```python
from build123d import *

# Parameters (mm, degrees)
SKETCH1_W           = 42
SKETCH1_H           = 14
SKETCH1_R           = 2.75
BOSS_EXTRUDE1_DEPTH = 12.7
SKETCH2_W           = 7
SKETCH2_H           = 1.27
CUT_EXTRUDE1_DEPTH  = 14


with BuildPart() as part:
    # Sketch1 → Boss-Extrude1 (new body)
    with BuildSketch(Plane(origin=(0, 0, 0), x_dir=(1, 0, 0), z_dir=(0, 1, 0))):
        Rectangle(SKETCH1_W, SKETCH1_H)
        with Locations((-16, 0)):
            Circle(SKETCH1_R, mode=Mode.SUBTRACT)
        with Locations((16, 0)):
            Circle(SKETCH1_R, mode=Mode.SUBTRACT)
    extrude(amount=BOSS_EXTRUDE1_DEPTH)

    # Sketch2 → Cut-Extrude1 (cut)
    with BuildSketch(Plane.XY.offset(7)):
        with Locations((0, 0.635)):
            Rectangle(SKETCH2_W, SKETCH2_H)
    extrude(amount=-CUT_EXTRUDE1_DEPTH, mode=Mode.SUBTRACT)


solid = part.part
```
The listing builds one solid part. Answer for the finished solid, in the listing's coordinates (mm). A direction names the side the tool comes from. Coordinates: 2 decimals unless noted, no trailing zeros. Loops run counter-clockwise (first coordinate to the right, second up) from the corner with the lowest first, then second, coordinate; pieces in that order, holes last. Notation, with made-up numbers: (-7, 40.25) -> (48, 40.25) arc R29 cw to (48, 75.25) -> close; hole circle Ø2 at (78, -22.75). An arc over 180 degrees is marked (long way). Use one line per item in the form item = value. Start each with the question number.
Item 1: Flat-ended cylindrical pins translate along their axes: pin 1 Ø3.5 at (x, z) = (1, -3.5) entering from -Y; pin 2 Ø7 at (x, z) = (16, 0) entering from +Y. Find the tip coordinate at first contact, or state that the pin passes through.
Item 2: The part is cut by section A-A on x = -16. Determine the outline of the cut face in (y, z), then the cut area to 3 significant figures.
Item 3: The part is cut by section C-C on y = 7.5. Determine the outline of the cut face in (x, z).
Item 4: A tool of negligible diameter and unlimited length cuts with its end or side. For faces 4 (the face through (13.253, 6.261, -0.121)), 5 (the face through (3.5, 1, 0)), from which of +Z, -Z, +X, -X, +Y, -Y can it reach the whole face along a straight path? Write none if from no direction.
Item 5: Consider L1, parallel to X at y = 9.5, z = 0; L2, parallel to Z at x = 16, y = 8; L3, parallel to Y at x = 2, z = -2.75. Determine where each line is inside the solid, lowest interval first. Write a range as [from, to].
Item 6: The part is cut by section D-D on z = -6. Determine the outline of the cut face in (x, y), then the cut area to 3 significant figures.
Item 7: The mould has two halves that part along X. Classify faces 1 (the face through (0, 1.27, 0)), 2 (the face through (-21, 6, 0)), 3 (the face through (21, 6, 0)): released by +X, released by -X, zero draft, split by the parting line, or undercut.
Item 8: The part is cut by section B-B on z = 0. Determine the outline of the cut face in (x, y), then the cut area to 3 significant figures.
Answer key:
q1.pin_1 = 1.27
q1.pin_2 = 12.7
q2.outline = (0, -7) -> (12.7, -7) -> (12.7, -2.75) -> (0, -2.75) -> close; (0, 2.75) -> (12.7, 2.75) -> (12.7, 7) -> (0, 7) -> close
q2.area = 108 mm2
q3.outline = (-21, -7) -> (21, -7) -> (21, 7) -> (-21, 7) -> close; hole circle Ø5.5 at (-16, 0); hole circle Ø5.5 at (16, 0)
q4.face_4 = +Y, -Y
q4.face_5 = +Z, -Z, -Y
q5.L1 = [-21, -18.75], [-13.25, 13.25], [18.75, 21]
q5.L2 = [-7, -2.75], [2.75, 7]
q5.L3 = [1.27, 12.7]
q6.outline = (-21, 0) -> (-3.5, 0) -> (-3.5, 1.27) -> (3.5, 1.27) -> (3.5, 0) -> (21, 0) -> (21, 12.7) -> (-21, 12.7) -> close
q6.area = 525 mm2
q7.face_1 = undercut
q7.face_2 = released by -X
q7.face_3 = released by +X
q8.outline = (-21, 0) -> (-18.75, 0) -> (-18.75, 12.7) -> (-21, 12.7) -> close; (-13.25, 0) -> (-3.5, 0) -> (-3.5, 1.27) -> (3.5, 1.27) -> (3.5, 0) -> (13.25, 0) -> (13.25, 12.7) -> (-13.25, 12.7) -> close; (18.75, 0) -> (21, 0) -> (21, 12.7) -> (18.75, 12.7) -> close
q8.area = 385 mm2
